Verification items for the finished model (mm, model axes). Give positions to 0.01 mm unless a question says otherwise; leave off trailing zeros. Loops run counter-clockwise (first coordinate to the right, second up) from the corner with the lowest first, then second, coordinate; pieces in that order, holes last. Notation, with made-up numbers: (-34, 53.25) - (-29, 53.25) arc R29 cw to (-29, 90.25) - close; hole circle Ø5 at (67.5, 30.5). An arc over 180 degrees is marked (long way). Answer in a Markdown table with one row per item.
```python
from build123d import *

# Parameters (mm, degrees)
SKETCH1_W           = 130
SKETCH1_H           = 130
SKETCH1_R           = 12.5
SKETCH1_R_2         = 4
BOSS_EXTRUDE1_DEPTH = 5
SKETCH2_R           = 3
CUT_EXTRUDE1_DEPTH  = 10
SKETCH3_R           = 3.5
CUT_EXTRUDE2_DEPTH  = 5


with BuildPart() as part:
    # Sketch1 → Boss-Extrude1 (new body)
    with BuildSketch(Plane(origin=(0, 0, 0), x_dir=(1, 0, 0), z_dir=(0, 1, 0))):
        Rectangle(SKETCH1_W, SKETCH1_H)
        with Locations(Location((0, 0, 0), (0, 0, 270))):
            Circle(SKETCH1_R, mode=Mode.SUBTRACT)
        with Locations(Location((-55, 0, 0), (0, 0, 270))):
            Circle(SKETCH1_R_2, mode=Mode.SUBTRACT)
        with Locations(Location((55, 0, 0), (0, 0, 270))):
            Circle(SKETCH1_R_2, mode=Mode.SUBTRACT)
    extrude(amount=BOSS_EXTRUDE1_DEPTH)

    # Sketch2 → Cut-Extrude1 (cut)
    with BuildSketch(Plane(origin=(0, 5, 0), x_dir=(1, 0, 0), z_dir=(0, 1, 0))):
        with Locations(Location((-25, 55, 0), (0, 0, 270))):
            Circle(SKETCH2_R)
        with Locations(Location((25, 55, 0), (0, 0, 270))):
            Circle(SKETCH2_R)
        with Locations(Location((25, -55, 0), (0, 0, 270))):
            Circle(SKETCH2_R)
        with Locations(Location((-25, -55, 0), (0, 0, 270))):
            Circle(SKETCH2_R)
    extrude(amount=-CUT_EXTRUDE1_DEPTH, mode=Mode.SUBTRACT)

    # Sketch3 → Cut-Extrude2 (cut)
    with BuildSketch(Plane(origin=(0, 5, 0), x_dir=(1, 0, 0), z_dir=(0, 1, 0))):
        with Locations(Location((-15.5, 15.5, 0), (0, 0, 270))):
            Circle(SKETCH3_R)
        with Locations(Location((15.5, 15.5, 0), (0, 0, 270))):
            Circle(SKETCH3_R)
        with Locations(Location((-15.5, -15.5, 0), (0, 0, 270))):
            Circle(SKETCH3_R)
        with Locations(Location((15.5, -15.5, 0), (0, 0, 270))):
            Circle(SKETCH3_R)
    extrude(amount=-CUT_EXTRUDE2_DEPTH, mode=Mode.SUBTRACT)


solid = part.part
```
Q1. Sectioned sample at C-C (z = 55). Record the cut outline in (x, y), and give its area (3 significant figures).
Completed:
| item | result |
|---|---|
| outline | (-65, 0) - (-28, 0) - (-28, 5) - (-65, 5) - close; (-22, 0) - (22, 0) - (22, 5) - (-22, 5) - close; (28, 0) - (65, 0) - (65, 5) - (28, 5) - close |
| area | 590 mm^2 |
Q2. Sectioned sample at D-D (x = -15.5). Record the cut outline in (y, z), and give its area (3 significant figures).
Completed:
| item | result |
|---|---|
| outline | (0, -65) - (5, -65) - (5, -19) - (0, -19) - close; (0, -12) - (5, -12) - (5, 12) - (0, 12) - close; (0, 19) - (5, 19) - (5, 65) - (0, 65) - close |
| area | 580 mm^2 |
Q3. Thickness scan on line 1 (X direction, y = 3.55, z = -55); line 2 (X direction, y = 3.2, z = 0); line 3 (Z direction, x = 14, y = 1.9). Record the ranges inside material, lowest first.
Completed:
| item | result |
|---|---|
| line 1 | -65 to -28, -22 to 22, 28 to 65 |
| line 2 | -65 to -59, -51 to -12.5, 12.5 to 51, 59 to 65 |
| line 3 | -65 to -18.66, -12.34 to 12.34, 18.66 to 65 |
Q4. Sectioned sample at B-B (x = 55). Record the cut outline in (y, z), and give its area (3 significant figures).
Completed:
| item | result |
|---|---|
| outline | (0, -65) - (5, -65) - (5, -4) - (0, -4) - close; (0, 4) - (5, 4) - (5, 65) - (0, 65) - close |
| area | 610 mm^2 |
Q5. Draft check along X on faces 1 (the face through (-65, 2, 1)), 2 (the face through (-25, 3, -58)), 3 (the face through (65, 2, 1)). Enter one of: +X half, -X half, draft (parallel to the pull), parting line (faces both ways), or undercut.
Completed:
| item | result |
|---|---|
| face 1 | -X half |
| face 2 | undercut |
| face 3 | +X half |
Q6. Sectioned sample at A-A (z = 0). Record the cut outline in (x, y).
Completed:
| item | result |
|---|---|
| outline | (-65, 0) - (-59, 0) - (-59, 5) - (-65, 5) - close; (-51, 0) - (-12.5, 0) - (-12.5, 5) - (-51, 5) - close; (12.5, 0) - (51, 0) - (51, 5) - (12.5, 5) - close; (59, 0) - (65, 0) - (65, 5) - (59, 5) - close |
